```python
from build123d import *

# Parameters (mm, degrees)
SKETCH_1_W          = 60
SKETCH_1_H          = 40
EXTRUDE_1_DEPTH     = 5
SKETCH_2_W          = 10
SKETCH_2_H          = 40
EXTRUDE_2_DEPTH     = 100
SKETCH_3_R          = 1
EXTRUDE_3_DEPTH     = 2.5
CUT_EXTRUDE_1_DEPTH = 11
SKETCH_5_W          = 5
SKETCH_5_H          = 50
CUT_EXTRUDE_2_DEPTH = 41
CUT_EXTRUDE_3_REACH = 7


with BuildPart() as part:
    # 草图1 → 凸台-拉伸1 (new body)
    with BuildSketch(Plane.XY):
        Rectangle(SKETCH_1_W, SKETCH_1_H)
    extrude(amount=EXTRUDE_1_DEPTH)

    # 草图2 → 凸台-拉伸2 (add)
    with BuildSketch(Plane.XY.offset(5)):
        with Locations((25, 0)):
            Rectangle(SKETCH_2_W, SKETCH_2_H)
    extrude(amount=EXTRUDE_2_DEPTH)

    # 草图3 → 凸台-拉伸3 (add)
    with BuildSketch(Plane.ZY.offset(-20)):
        with Locations((30, 0)):
            Circle(SKETCH_3_R)
    extrude(amount=EXTRUDE_3_DEPTH)

    # 草图4 → 切除-拉伸1 (cut, through all)
    with BuildSketch(Plane.ZY.offset(-20)):
        with BuildLine():
            Line((67, 6), (87, 6))
            ThreePointArc((87, 6), (88, 5), (87, 4))
            Line((87, 4), (67, 4))
            ThreePointArc((67, 4), (66, 5), (67, 6))
        make_face()
        with BuildLine():
            Line((67, -6), (87, -6))
            ThreePointArc((87, -6), (88, -5), (87, -4))
            Line((87, -4), (67, -4))
            ThreePointArc((67, -4), (66, -5), (67, -6))
        make_face()
    extrude(amount=-CUT_EXTRUDE_1_DEPTH, mode=Mode.SUBTRACT)

    # 草图5 → 切除-拉伸2 (cut, through all)
    with BuildSketch(Plane.XZ.offset(20)):
        with Locations((22.5, 80)):
            Rectangle(SKETCH_5_W, SKETCH_5_H)
    extrude(amount=-CUT_EXTRUDE_2_DEPTH, mode=Mode.SUBTRACT)

    # 草图6 → 切除-拉伸3 (cut, up to next)
    with BuildSketch(Plane.XY.offset(5), mode=Mode.PRIVATE) as cut_extrude_3_sk1:
        with BuildLine():
            Line((-11.5, 9.001468336), (-21.5, 9.001468336))
            ThreePointArc((-21.5, 9.001468336), (-22.498531664, 10), (-21.5, 10.998531664))
            Line((-21.5, 10.998531664), (-11.5, 10.998531664))
            ThreePointArc((-11.5, 10.998531664), (-10.501468336, 10), (-11.5, 9.001468336))
        make_face()
    cut_extrude_3_tool1 = extrude(cut_extrude_3_sk1.sketch, amount=-CUT_EXTRUDE_3_REACH, mode=Mode.PRIVATE) & part.part
    add(cut_extrude_3_tool1.solids().sort_by_distance((-16.5, 10, 5))[0], mode=Mode.SUBTRACT)
    # 草图6 → 切除-拉伸3 (cut, up to next)
    with BuildSketch(Plane.XY.offset(5), mode=Mode.PRIVATE) as cut_extrude_3_sk2:
        with BuildLine():
            Line((-11.5, -9.001468336), (-21.5, -9.001468336))
            ThreePointArc((-21.5, -9.001468336), (-22.498531664, -10), (-21.5, -10.998531664))
            Line((-21.5, -10.998531664), (-11.5, -10.998531664))
            ThreePointArc((-11.5, -10.998531664), (-10.501468336, -10), (-11.5, -9.001468336))
        make_face()
    cut_extrude_3_tool2 = extrude(cut_extrude_3_sk2.sketch, amount=-CUT_EXTRUDE_3_REACH, mode=Mode.PRIVATE) & part.part
    add(cut_extrude_3_tool2.solids().sort_by_distance((-16.5, -10, 5))[0], mode=Mode.SUBTRACT)


solid = part.part
```
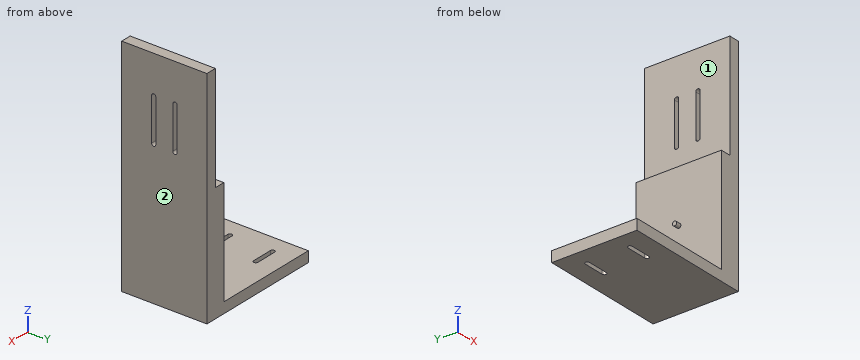
CAD build for the part. Positions are in the model's coordinates, mm. Face numbers are marked on the shaded views. A direction names the side the tool comes from. Coordinates: 2 decimals unless noted, no trailing zeros. Loops run counter-clockwise (first coordinate to the right, second up) from the corner with the lowest first, then second, coordinate; pieces in that order, holes last. Notation, with made-up numbers: (-5, 4.5) - (54, 4.5) arc R37 ccw to (54, 41.5) - close; hole circle Ø6 at (33, -28). An arc over 180 degrees is marked (long way). Return JSON: item names as keys, results as strings.
1. Band-saw the part on A-A (y = -14). Give the cut face in (x, z), and give its area (3 significant figures).
Result:
{"outline": "(-30, 0) - (30, 0) - (30, 105) - (25, 105) - (25, 55) - (20, 55) - (20, 5) - (-30, 5) - close", "area": "1,050 mm2"}
2. Band-saw the part on C-C (z = 94.5). Give the cut face in (x, y).
Result:
{"outline": "(25, -20) - (30, -20) - (30, 20) - (25, 20) - close"}
3. Probe L1, parallel to Y at x = 27.5, z = 68; L2, parallel to X at y = -4, z = 27.5; L3, parallel to Z at x = -7, y = 11.5. List the from-to ranges inside material, lowest first. Write a range as from..to.
Result:
{"L1": "y = -20..-6, -4..4, 6..20", "L2": "x = 20..30", "L3": "z = 0..5"}
4. Drop flat-ended pins along their axis: pin 1 (6 mm diameter, centred on y = 1, z = 87, fed in from -X); pin 2 (12 mm diameter, centred on x = 12, y = 12.5, fed in from +Z); pin 3 (1.6 mm diameter, centred on y = -0.5, z = 29.5, fed in from -X). Give the stop position or say it passes through.
Result:
{"pin 1": "stops at x = 25", "pin 2": "stops at z = 5", "pin 3": "stops at x = 17.5"}
5. Band-saw the part on B-B (x = -3). Give the cut face in (y, z).
Result:
{"outline": "(-20, 0) - (20, 0) - (20, 5) - (-20, 5) - close"}
6. 3-axis set-ups, long thin cutter, end or side, ignore diameter. For the marked faces 1 and 2: which of +Z, -Z, +X, -X, +Y, -Y reach the whole face in a straight line?
Result:
{"face 1": "+Z, -X, +Y, -Y", "face 2": "+Z, -Z, +X, +Y, -Y"}
